```python
from build123d import *

# Parameters (mm, degrees)
SKETCH1_W               = 8
SKETCH1_H               = 8
BOSS_EXTRUDE1_DEPTH     = 3
CUT_EXTRUDE1_DEPTH      = 12.704699911
CUT_EXTRUDE1_DEPTH_BACK = 12.704699911
CUT_EXTRUDE2_DEPTH      = 11
SKETCH4_R               = 1.75
CUT_EXTRUDE3_DEPTH      = 0.4
SKETCH5_W               = 8
SKETCH5_H               = 1
BOSS_EXTRUDE2_DEPTH     = 2
FILLET1_R               = 4
SKETCH6_W               = 4
SKETCH6_H               = 2.2
CUT_EXTRUDE4_DEPTH      = 0.4


with BuildPart() as part:
    # Sketch1 → Boss-Extrude1 (new body)
    with BuildSketch(Plane(origin=(0, 0, 0), x_dir=(1, 0, 0), z_dir=(0, 1, 0))):
        with Locations((4, 4)):
            Rectangle(SKETCH1_W, SKETCH1_H)
    extrude(amount=BOSS_EXTRUDE1_DEPTH)

    # Sketch2 → Cut-Extrude1 (cut, two sides: drawn at the far end of the back side and taken through both)
    with BuildSketch(Plane.XY.offset(-CUT_EXTRUDE1_DEPTH_BACK)):
        Polygon((0, 0), (0.6, 3), (0, 3), align=None)
        Polygon((8, 0), (7.4, 3), (8, 3), align=None)
    extrude(amount=CUT_EXTRUDE1_DEPTH + CUT_EXTRUDE1_DEPTH_BACK, mode=Mode.SUBTRACT)

    # Sketch3 → Cut-Extrude2 (cut)
    with BuildSketch(Plane(origin=(0, 0, 0), x_dir=(0, 0, -1), z_dir=(1, 0, 0))):
        Polygon((0, 0), (0.6, 3), (0, 3), align=None)
        Polygon((8, 3), (7.4, 3), (8, 0), align=None)
    extrude(amount=CUT_EXTRUDE2_DEPTH, mode=Mode.SUBTRACT)

    # Sketch4 → Cut-Extrude3 (cut)
    with BuildSketch(Plane.XZ):
        with Locations(Location((4, -3.75, 0), (0, 0, 270))):
            Circle(SKETCH4_R)
    extrude(amount=-CUT_EXTRUDE3_DEPTH, mode=Mode.SUBTRACT)

    # Sketch5 → Boss-Extrude2 (add)
    with BuildSketch(Plane.XZ):
        with Locations((4, -7.5)):
            Rectangle(SKETCH5_W, SKETCH5_H)
    extrude(amount=BOSS_EXTRUDE2_DEPTH)

    # Fillet1
    # the kernel refuses this fillet: 4 mm, written as the material it takes off along each edge
    with BuildSketch(Plane(origin=(8, -2, -16.660254038), x_dir=(0, 1, 0), z_dir=(0, 0, 1)), Plane(origin=(0, -2, 1.660254038), x_dir=(0, 1, 0), z_dir=(0, 0, -1))) as fillet1_piece_1:
        with BuildLine():
            CenterArc((4, 3.464101615), FILLET1_R, 180, 60)
            Line((0, 3.464101615), (-0.08, 3.464101615))
            Line((-0.08, 3.464101615), (-0.08, 0))
            Line((-0.08, 0), (0, -0.08))
            ThreePointArc((0, -0.08), (1, -0.08), (1.96, -0.069282032))
            Line((1.96, -0.069282032), (2, 0))
        make_face()
    extrude(amount=18.320508076, mode=Mode.SUBTRACT)

    # Sketch6 → Cut-Extrude4 (cut)
    with BuildSketch(Plane(origin=(0, 3, 0), x_dir=(1, 0, 0), z_dir=(0, 1, 0))):
        with Locations((3, 4)):
            Rectangle(SKETCH6_W, SKETCH6_H)
        Polygon((5, 2), (5, 2.9), (5, 5.1), (5, 6), (7, 4), align=None)
    extrude(amount=-CUT_EXTRUDE4_DEPTH, mode=Mode.SUBTRACT)


solid = part.part
```
Check sheet for the modelled part. Datum: model origin and axes. Units: mm. A direction names the side the tool comes from. Give positions to 0.01 mm unless a question says otherwise; leave off trailing zeros. Loops run counter-clockwise (first coordinate to the right, second up) from the corner with the lowest first, then second, coordinate; pieces in that order, holes last. Notation, with made-up numbers: (85.5, -12.5) - (141.5, -12.5) arc R14 ccw to (141.5, 13.5) - close; hole circle Ø3 at (15, -39). An arc over 180 degrees is marked (long way). One line per question, with ' | ' between items. Start each with the question number.
1. Gauge pin test, flat ends, axial feed: pin 1 Ø1.5 at (x, z) = (6, -3) entering from -Y; pin 2 Ø1 at (x, y) = (1.5, -1) entering from +Z; pin 3 Ø1.5 at (y, z) = (1, -6.5) entering from -X. Record the tip position at first contact, or that the pin passes through.
2. Cross-section at B-B, the plane x = 4. Enter the section's corners in (y, z), plus the area to 3 significant figures.
3. Draft check along X on faces 4 (the flat face through (3, 0, -2)), 5 (the flat face through (4, 2.6, -4)), 6 (the cylindrical face through (1.49, -1.48, -7.49)). Enter one of: released by +X, released by -X, zero draft, split by the parting line, or undercut.
4. Cross-section at C-C, the plane y = 1.4. Enter the section's corners in (x, z).
5. Cross-section at D-D, the plane z = -3.75. Enter the section's corners in (x, y), plus the area to 3 significant figures.
6. Material ranges on line 1 along Z through (x, y) = (5.25, -0.15); line 2 along Y through (x, z) = (2.25, -4.75); line 3 along X through (y, z) = (0.1, -3.75), recorded low to high. Write a range as [from, to].
7. Cross-section at A-A, the plane z = -7.25. Enter the section's corners in (x, y).
8. Set-up check for faces 1 (the cylindrical face through (2.94, 0.2, -2.36)), 2 (the flat face through (4, -1, -7)), 3 (the flat face through (6, 2.8, -5)): record each of +Z, -Z, +X, -X, +Y, -Y from which the full face is reachable in a straight line by a thin tool's end or side.
Check result:
1) pin 1: stops at y = 0 | pin 2: stops at z = -7 | pin 3: stops at x = 0.05
2) outline: (-2, -8) - (0, -8) - (3, -7.4) - (3, -5.1) - (2.6, -5.1) - (2.6, -2.9) - (3, -2.9) - (3, -0.6) - (0, 0) - (0, -2) - (0.4, -2) - (0.4, -5.5) - (0, -5.5) - (0, -7) - (-2, -7) - close | area: 21.9 mm2
3) face 4: zero draft | face 5: undercut | face 6: released by -X
4) outline: (0.28, -7.72) - (7.72, -7.72) - (7.72, -0.28) - (0.28, -0.28) - close
5) outline: (0, 0) - (2.25, 0) - (2.25, 0.4) - (5.75, 0.4) - (5.75, 0) - (8, 0) - (7.4, 3) - (6.75, 3) - (6.75, 2.6) - (1, 2.6) - (1, 3) - (0.6, 3) - close | area: 18.5 mm2
6) line 1: z = [-8, -7] | line 2: y = [0, 2.6] | line 3: x = [0.02, 2.25], [5.75, 7.98]
7) outline: (0, 0) arc R4 ccw to (3.46, -2) - (4.54, -2) arc R4 ccw to (8, 0) - (7.4, 3) - (0.6, 3) - close
8) face 1: -Y | face 2: +Z, +X, -X, -Y | face 3: +Y
